Geometry check sheet. Reference: the model listing, model coordinates, mm. A direction names the side the tool comes from. Give positions to 0.01 mm unless a question says otherwise; leave off trailing zeros. Order: outer loops, then holes, each group sorted by start corner. A loop starts at its lowest first (then second) coordinate and runs counter-clockwise, first axis right, second up. Notation, with made-up numbers: M 70.5,28.5 L 120.5,28.5 A19 cw 120.5,50.5 Z; hole C 27.5,11.25 d5. An arc over 180 degrees is marked long. Put each result on its own line as item: value. Start each with the question number.
Q1. Mould release check, pull along Y, two halves, no side actions. Record for faces 1 (the flat face through (-92, -126.95, -9)), 2 (the flat face through (-1, -133.5, 3)), 3 (the flat face through (-1, 2, 8)): +Y half, -Y half, draft (parallel to the pull), parting line (faces both ways), or undercut.
Q2. Section check C-C on y = 54.5. Record the cut outline in (x, z).
Q3. Section check B-B on x = -67. Record the cut outline in (y, z).
Q4. Section check A-A on z = -5.5. Record the cut outline in (x, y), then the cut area to 3 significant figures.
Q5. Access from +Z, -Z, +X, -X, +Y, -Y to the whole of each face (thin tool, end or side, straight path). Record for faces 4 (the flat face through (92, 126.95, -9)), 5 (the flat face through (-100.95, -30, -1)), 6 (the flat face through (-7, -130.95, -1)), 7 (the flat face through (-7, 130.95, -1)), 8 (the flat face through (100.95, -30, -1)).
Q6. Go/stop test with flat-tipped pins: pin 1 (1.1 mm diameter, centred on y = 126.5, z = -7, fed in from +X); pin 2 (1.2 mm diameter, centred on y = 128.5, z = -14, fed in from -X); pin 3 (4 mm diameter, centred on x = 20, y = 113.95, fed in from -Z); pin 4 (5 mm diameter, centred on x = 63, y = 86, fed in from -Z). Record where each tip stops, or that it passes through.
Q7. Material ranges on L1, parallel to Y at x = 20, z = 2.75; L2, parallel to Y at x = 89, z = -6.5; L3, parallel to Z at x = 41, y = -102, recorded low to high.
```python
from build123d import *

# Parameters (mm, degrees)
SKETCH1_W                                = 207
SKETCH1_H                                = 267
BOSS_EXTRUDE1_DEPTH                      = 8
SKETCH2_W                                = 201.9
SKETCH2_H                                = 261.9
BOSS_EXTRUDE2_DEPTH                      = 2
BOSS_EXTRUDE3_DEPTH                      = 14
CUT_EXTRUDE1_DEPTH                       = 281.717745253
MIRROR1_AT_THE_SECOND_PLANE_COPY_1_DEPTH = 14
MIRROR1_AT_THE_SECOND_PLANE_COPY_2_DEPTH = 281.717745253
SKETCH5_R                                = 2.1
CUT_EXTRUDE2_DEPTH                       = 170.500737462
CHAMFER1_SIZE                            = 2


with BuildPart() as part:
    # Sketch1 → Boss-Extrude1 (new body)
    with BuildSketch(Plane.XY):
        Rectangle(SKETCH1_W, SKETCH1_H)
    extrude(amount=BOSS_EXTRUDE1_DEPTH)

    # Sketch2 → Boss-Extrude2 (add)
    with BuildSketch(Plane(origin=(0, 0, 0), x_dir=(-1, 0, 0), z_dir=(0, 0, -1))):
        Rectangle(SKETCH2_W, SKETCH2_H)
    extrude(amount=BOSS_EXTRUDE2_DEPTH)

    # Sketch3 → Boss-Extrude3 (add)
    with BuildSketch(Plane(origin=(0, 0, -2), x_dir=(-1, 0, 0), z_dir=(0, 0, -1))):
        Polygon((86.95, -130.95), (86.95, -126.95), (96.95, -126.95), (96.95, -125.95), (100.95, -125.95), (100.95, -130.95), align=None)
    boss_extrude3 = extrude(amount=BOSS_EXTRUDE3_DEPTH)

    # Sketch4 → Cut-Extrude1 (cut, through all)
    with BuildSketch(Plane(origin=(0, -126.95, 0), x_dir=(1, 0, 0), z_dir=(0, 1, 0))):
        with BuildLine():
            Line((-89.85, 16), (-89.85, 12))
            ThreePointArc((-89.85, 12), (-91.95, 9.9), (-94.05, 12))
            Line((-94.05, 12), (-94.05, 16))
            ThreePointArc((-94.05, 16), (-91.95, 18.1), (-89.85, 16))
        make_face()
    cut_extrude1 = extrude(amount=-CUT_EXTRUDE1_DEPTH, mode=Mode.SUBTRACT)

    # Mirror1: Boss-Extrude3, Cut-Extrude1 across plane
    add(boss_extrude3.mirror(Plane.ZX))
    add(cut_extrude1.mirror(Plane.ZX), mode=Mode.SUBTRACT)

    # Mirror1 at the second plane: Boss-Extrude3, Cut-Extrude1 across plane
    add(boss_extrude3.mirror(Plane(origin=(0, 0, 0), x_dir=(0, 0, 1), z_dir=(1, 0, 0))))
    add(cut_extrude1.mirror(Plane(origin=(0, 0, 0), x_dir=(0, 0, 1), z_dir=(1, 0, 0))), mode=Mode.SUBTRACT)

    # Mirror1 at the second plane copy 1 sketc → Mirror1 at the second plane copy 1 (add)
    with BuildSketch(Plane(origin=(0, 0, -2), x_dir=(1, 0, 0), z_dir=(0, 0, -1))):
        Polygon((86.95, -130.95), (86.95, -126.95), (96.95, -126.95), (96.95, -125.95), (100.95, -125.95), (100.95, -130.95), align=None)
    extrude(amount=MIRROR1_AT_THE_SECOND_PLANE_COPY_1_DEPTH)

    # Mirror1 at the second plane copy 2 sketc → Mirror1 at the second plane copy 2 (cut, through all)
    with BuildSketch(Plane(origin=(0, 126.95, 0), x_dir=(-1, 0, 0), z_dir=(0, -1, 0))):
        with BuildLine():
            Line((-89.85, 16), (-89.85, 12))
            ThreePointArc((-89.85, 12), (-91.95, 9.9), (-94.05, 12))
            Line((-94.05, 12), (-94.05, 16))
            ThreePointArc((-94.05, 16), (-91.95, 18.1), (-89.85, 16))
        make_face()
    extrude(amount=-MIRROR1_AT_THE_SECOND_PLANE_COPY_2_DEPTH, mode=Mode.SUBTRACT)

    # Sketch5 → Cut-Extrude2 (cut, through all)
    with BuildSketch(Plane(origin=(0, 0, -2), x_dir=(-1, 0, 0), z_dir=(0, 0, -1))):
        with Locations((-20, 113.95)):
            Circle(SKETCH5_R)
        with Locations((20, 113.95)):
            Circle(SKETCH5_R)
    extrude(amount=-CUT_EXTRUDE2_DEPTH, mode=Mode.SUBTRACT)

    # Chamfer1
    chamfer1_edges = [part.edges().sort_by_distance(p)[0] for p in [
        (-103.5, 0, 8),
        (0, -133.5, 8),
        (103.5, 0, 8),
        (0, 133.5, 8),
    ]]
    chamfer(chamfer1_edges, length=CHAMFER1_SIZE)


solid = part.part
```
Results found:
1. face 1: undercut
1. face 2: -Y half
1. face 3: draft
2. outline: M -103.5,0 L -100.95,0 L -100.95,-2 L 100.95,-2 L 100.95,0 L 103.5,0 L 103.5,6 L 101.5,8 L -101.5,8 L -103.5,6 Z
3. outline: M -133.5,0 L -130.95,0 L -130.95,-2 L 130.95,-2 L 130.95,0 L 133.5,0 L 133.5,6 L 131.5,8 L -131.5,8 L -133.5,6 Z
4. outline: M -100.95,-130.95 L -86.95,-130.95 L -86.95,-126.95 L -96.95,-126.95 L -96.95,-125.95 L -100.95,-125.95 Z; M -100.95,125.95 L -96.95,125.95 L -96.95,126.95 L -86.95,126.95 L -86.95,130.95 L -100.95,130.95 Z; M 86.95,-130.95 L 100.95,-130.95 L 100.95,-125.95 L 96.95,-125.95 L 96.95,-126.95 L 86.95,-126.95 Z; M 86.95,126.95 L 96.95,126.95 L 96.95,125.95 L 100.95,125.95 L 100.95,130.95 L 86.95,130.95 Z
4. area: 240 mm^2
5. face 4: -Z
5. face 5: -Z, -X, +Y, -Y
5. face 6: -Z, +X, -X, -Y
5. face 7: -Z, +X, -X, +Y
5. face 8: -Z, +X, +Y, -Y
6. pin 1: stops at x = 100.95
6. pin 2: stops at x = -100.95
6. pin 3: passes through
6. pin 4: stops at z = -2
7. L1: y = -133.5 to 111.85, 116.05 to 133.5
7. L2: y = -130.95 to -126.95, 126.95 to 130.95
7. L3: z = -2 to 8
